The listing builds one solid part. Answer for the finished solid, in the listing's coordinates (mm). A direction names the side the tool comes from. Round coordinates to 2 decimals unless told otherwise and drop trailing zeros. Write each loop counter-clockwise with the first axis right and the second up, starting at its lowest first coordinate (ties: lowest second). Pieces come first, ordered by that corner, then holes. Notation, with made-up numbers: (61, 67) - (95, 67) arc R25 cw to (95, 97) - close; hole circle Ø7 at (38.25, 73). An arc over 180 degrees is marked (long way). Use a Markdown table: item, result. Add a question column.
1) Each of these flat-tipped pins is pushed along its axis until it touches: P1, Ø1, axis at x = -1, z = -25, coming from the -Y side; P2, Ø1, axis at y = 146.5, z = 7.5, coming from the +X side; P3, Ø4, axis at x = -22.5, z = -4.5, coming from the -Y side. Where does it stop, or does it pass through?
2) Find the intervals of material crossed by probe 1 along X at (y, z) = (73.5, -26); probe 2 along Z at (x, y) = (-27, 152); probe 3 along Y at (x, z) = (-10, 25.5), in increasing order. Write a range as from..to.
3) A cutting plane is placed at B-B (y = 76). Give the vertices of the cut face in (x, z).
4) A cutting plane is placed at C-C (x = -33). Give the vertices of the cut face in (y, z), then the cut area to 3 significant figures.
5) A cutting plane is placed at D-D (z = -25.5). Give the vertices of the cut face in (x, y).
6) A cutting plane is placed at A-A (z = 20). Give the vertices of the cut face in (x, y), then the cut area to 3 significant figures.
7) A tool of negligible diameter and unlimited length cuts with its end or side. For faces 1 (the flat face through (-20, 180, 0)), 2 (the flat face through (-38, 123, 0)), from which of +Z, -Z, +X, -X, +Y, -Y can it reach the whole face along a straight path? Write none if from no direction.
8) Determine the mould class of faces 3 (the flat face through (-20, 89, -30)), 4 (the flat face through (-40, 129, 0)), 5 (the flat face through (-19, 178, 0)) for opening direction Z: +Z half, -Z half, draft (parallel to the pull), parting line (faces both ways), or undercut.
Autodesk Inventor part; units mm, degrees
ref_plane "YZ Plane" through (0, 0, 0) normal (1, 0, 0) x (0, 1, 0)
ref_plane "XZ Plane" through (0, 0, 0) normal (0, 1, 0) x (-1, 0, 0)
ref_plane "XY Plane" through (0, 0, 0) normal (0, 0, 1) x (1, 0, 0)
sketch "Sketch1" plane through (0, 0, 0) normal (0, 1, 0) x (-1, 0, 0)
  line L0 (0, -28) -> (38, -28)
  line L1 (38, -28) -> (38, 28)
  line L2 (38, 28) -> (0, 28)
  line L3 (0, 28) -> (0, -28) construction
  line L4 (0, 30) -> (40, 30)
  line L5 (40, 30) -> (40, -30)
  line L6 (40, -30) -> (0, -30)
  line L7 (0, 30) -> (0, 28)
  line L8 (0, -28) -> (0, -30)
  point P0 (0, 0)
  point P1 (0, 0)
  dimension "d0" = 40
  dimension "d1" = 60
  dimension "d2" = 2
  dimension "d3" = 38
extrude "Extrusion1" add sketch "Sketch1" along normal blind 180
sketch "Sketch2" plane through (0, 180, 0) normal (0, 1, 0) x (1, 0, 0)
  line L0 (-38, 28) -> (0, 28)
  line L1 (0, -30) -> (0, -28)
  line L2 (-38, 28) -> (0, 28)
  line L3 (0, 28) -> (0, -28)
  line L4 (0, -28) -> (-38, -28)
  line L5 (-38, -28) -> (-38, 28)
  point P0 (0, 0)
extrude "Extrusion2" add sketch "Sketch2" against normal blind 2
sketch "Sketch3" plane through (-38, 0, -28) normal (0, 0, 1) x (1, 0, 0)
  line L0 (38, 178) -> (36, 178)
  line L1 (36, 178) -> (36, 128)
  line L2 (36, 128) -> (38, 128)
  line L3 (38, 128) -> (38, 178)
  point P0 (38, 0)
  dimension "d8" = 2
  dimension "d9" = 50
extrude "Extrusion3" add sketch "Sketch3" along normal blind 5
mirror "Mirror1" about plane through (0, 0, 0) normal (0, 0, 1) of "Extrusion3"
sketch "Sketch4" plane through (-38, 0, 28) normal (1, 0, 0) x (0, 0, -1)
  line L0 (0, 0) -> (56, 0)
  line L1 (56, 0) -> (56, 178)
  line L2 (0, 0) -> (56, 0)
  line L3 (56, 0) -> (56, 70)
  line L4 (56, 70) -> (0, 70)
  line L5 (0, 70) -> (0, 0)
  point P0 (28, 0)
  dimension "d12" = 70
extrude "Extrusion4" cut sketch "Sketch4" against normal blind 5
sketch "Sketch5" plane through (0, 0, -30) normal (1, 0, 0) x (0, 0, -1)
  line L0 (-2, 70) -> (-58, 70)
  line L1 (-2, 0) -> (-2, 128)
  line L2 (-58, 70) -> (-2, 70)
  line L3 (-2, 70) -> (-2, 80)
  line L4 (-2, 80) -> (-58, 80)
  line L5 (-58, 80) -> (-58, 70)
  point P0 (-30, 0)
  dimension "d15" = 10
extrude "Extrusion5" add sketch "Sketch5" against normal blind 2
properties part number "Soporte_camara"
Entries:
| question | item | result |
|---|---|---|
| 1 | P1 | stops at y = 70 |
| 1 | P2 | stops at x = -38 |
| 1 | P3 | stops at y = 178 |
| 2 | probe 1 | x = -40..-38, -2..0 |
| 2 | probe 2 | z = -30..-28, 28..30 |
| 2 | probe 3 | y = 178..180 |
| 3 | outline | (-40, -30) - (0, -30) - (0, 30) - (-40, 30) - close; hole (-38, -28) - (-2, -28) - (-2, 28) - (-38, 28) - close |
| 4 | outline | (0, -30) - (180, -30) - (180, 30) - (0, 30) - (0, 28) - (178, 28) - (178, -28) - (0, -28) - close |
| 4 | area | 832 mm² |
| 5 | outline | (-40, 70) - (-38, 70) - (-38, 178) - (-2, 178) - (-2, 128) - (0, 128) - (0, 180) - (-40, 180) - close; (-2, 70) - (0, 70) - (0, 80) - (-2, 80) - close |
| 6 | outline | (-40, 70) - (-38, 70) - (-38, 178) - (0, 178) - (0, 180) - (-40, 180) - close; (-2, 70) - (0, 70) - (0, 80) - (-2, 80) - close |
| 6 | area | 316 mm² |
| 7 | face 1 | +Z, -Z, +X, -X, +Y |
| 7 | face 2 | -Y |
| 8 | face 3 | -Z half |
| 8 | face 4 | draft |
| 8 | face 5 | undercut |
